Work out the finished part from the listing and answer in its coordinate system (mm). Round coordinates to 2 decimals unless told otherwise and drop trailing zeros. Write each loop counter-clockwise with the first axis right and the second up, starting at its lowest first coordinate (ties: lowest second). Pieces come first, ordered by that corner, then holes. Notation, with made-up numbers: M 55.25,56 L 63.25,56 A21 cw 63.25,92 Z; hole C 1.5,44 d11. An arc over 180 degrees is marked long. Answer in a Markdown table with one row per item.
```python
from build123d import *

# Parameters (mm, degrees)
SKETCH_1_R      = 1.5
SKETCH_1_W      = 14.999960721
SKETCH_1_H      = 6.000098196
SKETCH_1_H_2    = 6.000098195
SKETCH_1_W_2    = 14.999960722
EXTRUDE_1_DEPTH = 6


with BuildPart() as part:
    # Эскиз1 → Бобышка-Вытянуть1 (new body)
    with BuildSketch(Plane(origin=(0, 0, 0), x_dir=(1, 0, 0), z_dir=(0, 1, 0))):
        Polygon((-102.768102854, -104.532435011), (-102.768102854, -92.192478988), (-102.768102854, -82.192478988), (-102.768102854, 85.127608967), (-102.768102854, 95.127608967), (-102.768102854, 107.467564989), (-102.768102854, 112.467564989), (-97.768102854, 112.467564989), (114.231897146, 112.467564989), (119.231897146, 112.467564989), (119.231897146, 107.467564989), (119.231897146, -104.532435011), (119.231897146, -109.532435011), (114.231897146, -109.532435011), (-97.768102854, -109.532435011), (-102.768102854, -109.532435011), align=None)
        with Locations((-96.268102854, 105.967564989)):
            Circle(SKETCH_1_R, mode=Mode.SUBTRACT)
        with Locations((112.731897146, 105.967564989)):
            Circle(SKETCH_1_R, mode=Mode.SUBTRACT)
        with Locations((-96.268102854, -103.032435011)):
            Circle(SKETCH_1_R, mode=Mode.SUBTRACT)
        with Locations((112.731897146, -103.032435011)):
            Circle(SKETCH_1_R, mode=Mode.SUBTRACT)
        with Locations((103.231897146, 7.467564989)):
            Circle(SKETCH_1_R, mode=Mode.SUBTRACT)
        with Locations((113.231897146, 7.467564989)):
            Circle(SKETCH_1_R, mode=Mode.SUBTRACT)
        with Locations((113.231897146, -4.532435011)):
            Circle(SKETCH_1_R, mode=Mode.SUBTRACT)
        with Locations((103.231897146, -4.532435011)):
            Circle(SKETCH_1_R, mode=Mode.SUBTRACT)
        with Locations((-68.539568551, 105.467614087)):
            Rectangle(SKETCH_1_W, SKETCH_1_H, mode=Mode.SUBTRACT)
        with Locations((-68.539568551, -102.532484109)):
            Rectangle(SKETCH_1_W, SKETCH_1_H_2, mode=Mode.SUBTRACT)
        with BuildLine():
            Line((-15.30363676, 5.003098895), (-63.336645349, 53.036107484))
            Line((-63.336645349, 53.036107484), (-82.344918946, 72.044381082))
            ThreePointArc((-82.344918946, 72.044381082), (-87.793870014, 73.128244838), (-90.880452852, 68.508847176))
            Line((-90.880452852, 68.508847176), (-90.880452852, -65.573717197))
            ThreePointArc((-90.880452852, -65.573717197), (-87.793870014, -70.193114859), (-82.344918946, -69.109251103))
            Line((-82.344918946, -69.109251103), (-63.336645349, -50.100977505))
            Line((-63.336645349, -50.100977505), (-15.30363676, -2.067968916))
            ThreePointArc((-15.30363676, -2.067968916), (-13.839170666, 1.467564989), (-15.30363676, 5.003098895))
        make_face(mode=Mode.SUBTRACT)
        with BuildLine():
            Line((31.767431052, 5.003098895), (79.800439641, 53.036107484))
            ThreePointArc((79.800439641, 53.036107484), (85.249390708, 54.119971241), (88.335973547, 49.500573578))
            Line((88.335973547, 49.500573578), (88.335973547, -46.5654436))
            ThreePointArc((88.335973547, -46.5654436), (85.249390708, -51.184841262), (79.800439641, -50.100977505))
            Line((79.800439641, -50.100977505), (31.767431052, -2.067968916))
            ThreePointArc((31.767431052, -2.067968916), (30.302964958, 1.467564989), (31.767431052, 5.003098895))
        make_face(mode=Mode.SUBTRACT)
        with BuildLine():
            Line((4.69636324, 25.003098895), (-43.336645349, 73.036107484))
            Line((-43.336645349, 73.036107484), (-56.892612926, 86.592075061))
            ThreePointArc((-56.892612926, 86.592075061), (-57.976476682, 92.041026129), (-53.35707902, 95.127608967))
            Line((-53.35707902, 95.127608967), (69.820873311, 95.127608967))
            ThreePointArc((69.820873311, 95.127608967), (74.440270974, 92.041026129), (73.356407217, 86.592075061))
            Line((73.356407217, 86.592075061), (59.800439641, 73.036107484))
            Line((59.800439641, 73.036107484), (11.767431052, 25.003098895))
            ThreePointArc((11.767431052, 25.003098895), (8.231897146, 23.538632801), (4.69636324, 25.003098895))
        make_face(mode=Mode.SUBTRACT)
        with BuildLine():
            Line((69.820873311, -92.192478988), (-53.35707902, -92.192478988))
            ThreePointArc((-53.35707902, -92.192478988), (-57.976476682, -89.10589615), (-56.892612926, -83.656945082))
            Line((-56.892612926, -83.656945082), (-43.336645349, -70.100977505))
            Line((-43.336645349, -70.100977505), (4.69636324, -22.067968916))
            ThreePointArc((4.69636324, -22.067968916), (8.231897146, -20.603502822), (11.767431052, -22.067968916))
            Line((11.767431052, -22.067968916), (59.800439641, -70.100977505))
            Line((59.800439641, -70.100977505), (73.356407217, -83.656945082))
            ThreePointArc((73.356407217, -83.656945082), (74.440270974, -89.10589615), (69.820873311, -92.192478988))
        make_face(mode=Mode.SUBTRACT)
        with Locations((85.003362843, -102.532484109)):
            Rectangle(SKETCH_1_W_2, SKETCH_1_H_2, mode=Mode.SUBTRACT)
        with Locations((85.003362843, 105.467614087)):
            Rectangle(SKETCH_1_W_2, SKETCH_1_H, mode=Mode.SUBTRACT)
    extrude(amount=EXTRUDE_1_DEPTH)


solid = part.part
```
1. The part is cut by section A-A (z = -91). Determine the outline of the cut face in (x, y), plus the area to 3 significant figures.
Calculated:
| item | result |
|---|---|
| outline | M -102.77,0 L -58.28,0 L -58.28,6 L -102.77,6 Z; M 74.74,0 L 119.23,0 L 119.23,6 L 74.74,6 Z |
| area | 534 mm² |
2. Determine the mould class of faces 1 (the flat face through (10, 3, -112.468)), 2 (the flat face through (7, 3, -95.128)), 3 (the flat face through (7, 3, 109.532)) for opening direction Z: released by +Z, released by -Z, zero draft, split by the parting line, or undercut.
Calculated:
| item | result |
|---|---|
| face 1 | released by -Z |
| face 2 | undercut |
| face 3 | released by +Z |
3. The part is cut by section B-B (x = -66.5). Determine the outline of the cut face in (y, z), plus the area to 3 significant figures.
Calculated:
| item | result |
|---|---|
| outline | M 0,-112.47 L 6,-112.47 L 6,-108.47 L 0,-108.47 Z; M 0,-102.47 L 6,-102.47 L 6,-56.2 L 0,-56.2 Z; M 0,53.26 L 6,53.26 L 6,99.53 L 0,99.53 Z; M 0,105.53 L 6,105.53 L 6,109.53 L 0,109.53 Z |
| area | 603 mm² |
4. Consider line 1 along X through (y, z) = (5.2, -103); line 2 along X through (y, z) = (2, 36); line 3 along X through (y, z) = (3.15, 57). Determine where each line is inside the solid, lowest interval first. Write a range as from..to.
Calculated:
| item | result |
|---|---|
| line 1 | x = -102.77..-76.04, -61.04..77.5, 92.5..119.23 |
| line 2 | x = -102.77..-90.88, -49.24..-9.24, 25.7..65.7, 88.34..119.23 |
| line 3 | x = -102.77..-90.88, -70.24..-30.24, 46.7..119.23 |
5. The part is cut by section C-C (x = 8). Determine the outline of the cut face in (y, z).
Calculated:
| item | result |
|---|---|
| outline | M 0,-112.47 L 6,-112.47 L 6,-95.13 L 0,-95.13 Z; M 0,-23.54 L 6,-23.54 L 6,20.61 L 0,20.61 Z; M 0,92.19 L 6,92.19 L 6,109.53 L 0,109.53 Z |
6. The part is cut by section D-D (z = 32.5). Determine the outline of the cut face in (x, y), plus the area to 3 significant figures.
Calculated:
| item | result |
|---|---|
| outline | M -102.77,0 L -90.88,0 L -90.88,6 L -102.77,6 Z; M -45.74,0 L -5.74,0 L -5.74,6 L -45.74,6 Z; M 22.2,0 L 62.2,0 L 62.2,6 L 22.2,6 Z; M 88.34,0 L 119.23,0 L 119.23,6 L 88.34,6 Z |
| area | 737 mm² |
